Source: CAD feature listing. Evaluate the final solid. Frame: model axes, mm. A direction names the side the tool comes from. Round coordinates to 2 decimals unless told otherwise and drop trailing zeros. Write each loop counter-clockwise with the first axis right and the second up, starting at its lowest first coordinate (ties: lowest second). Pieces come first, ordered by that corner, then holes.
Autodesk Fusion 360 part; units mm, degrees
sketch "Sketch1" plane through (0, 0, 0) normal (0, 0, 1) x (1, 0, 0)
  line L0 (-42.9734, 5.15) -> (-45.9467, 0)
  line L1 (-45.9467, 0) -> (-42.9734, -5.15)
  line L2 (-42.9734, -5.15) -> (-37.0266, -5.15)
  line L3 (-37.0266, -5.15) -> (-34.0533, 0)
  line L4 (-34.0533, 0) -> (-37.0266, 5.15)
  line L5 (-37.0266, 5.15) -> (-42.9734, 5.15)
  line L6 (46, 5.15) -> (34, 5.15)
  line L7 (34, 5.15) -> (34, -5.15)
  line L8 (34, -5.15) -> (46, -5.15)
  line L9 (46, 5.15) -> (34, -5.15) construction
  line L10 (34, 5.15) -> (46, -5.15) construction
  line L11 (-32.8586, 7) -> (22.9763, 7)
  arc A0 (-32.8586, 7) -> (-32.8586, -7) centre (-40, 0) ccw
  arc A1 (22.9763, -7) -> (46, -5.15) centre (34, 0) ccw
  arc A2 (46, 5.15) -> (22.9763, 7) centre (34, 0) ccw
  line L12 (-32.8586, -7) -> (22.9763, -7)
  point P0 (-40, 0)
  point P1 (40, 0)
  dimension "d1" = 80
  dimension "d2" = 5.15
  dimension "d3" = 20
  dimension "d4" = 12
  dimension "d5" = 10.3
sketch "Sketch2" plane through (0, 0, 0) normal (0, 0, 1) x (1, 0, 0)
extrude "Extrude1" add sketch "Sketch1" along normal blind 4
fillet "Fillet1" radius 5 4 edges at (-32.8586, -7, 2) (22.9763, -7, 2) (22.9763, 7, 2) (-32.8586, 7, 2)
sketch "Sketch3" plane through (0, 0, 4) normal (0, 0, 1) x (1, 0, 0)
  line L0 (-42.9734, 5.15) -> (-37.0266, 5.15)
  line L1 (-37.0266, 5.15) -> (-34.0533, 0)
  line L2 (-34.0533, 0) -> (-37.0266, -5.15)
  line L3 (-37.0266, -5.15) -> (-42.9734, -5.15)
  line L4 (-42.9734, -5.15) -> (-45.9467, 0)
  line L5 (-45.9467, 0) -> (-42.9734, 5.15)
  arc A0 (-34, 8) -> (-34, -8) centre (-40, 0) ccw
  arc A1 (-31, -7) -> (-34, -8) centre (-31, -12) ccw
  line L6 (-31, -7) -> (20.5053, -7)
  arc A2 (24.2417, -8.6775) -> (20.5053, -7) centre (20.5053, -12) ccw
  arc A3 (24.2417, -8.6775) -> (46, -5.15) centre (34, 0) ccw
  line L7 (46, -5.15) -> (34, -5.15)
  line L8 (34, -5.15) -> (34, 5.15)
  line L9 (34, 5.15) -> (46, 5.15)
  arc A4 (46, 5.15) -> (24.2417, 8.6775) centre (34, 0) ccw
  arc A5 (20.5053, 7) -> (24.2417, 8.6775) centre (20.5053, 12) ccw
  line L10 (20.5053, 7) -> (-31, 7)
  arc A6 (-34, 8) -> (-31, 7) centre (-31, 12) ccw
  line L11 (-22.5, 2.5) -> (22.5, 2.5)
  line L12 (22.5, 2.5) -> (22.5, -2.5)
  line L13 (22.5, -2.5) -> (-22.5, -2.5)
  line L14 (-22.5, -2.5) -> (-22.5, 2.5)
  line L15 (-22.5, 2.5) -> (22.5, -2.5) construction
  line L16 (22.5, 2.5) -> (-22.5, -2.5) construction
  dimension "d11" = 45
  dimension "d12" = 5
extrude "Extrude2" cut sketch "Sketch3" against normal blind 1 contours L11 L12 L13 L14
sketch "Sketch4" plane through (0, 0, 4) normal (0, 0, 1) x (1, 0, 0)
  line L0 (22.5, 2.5) -> (22.5, -2.5)
  line L1 (22.5, -2.5) -> (-22.5, -2.5)
  line L2 (-22.5, -2.5) -> (-22.5, 2.5)
  line L3 (-22.5, 2.5) -> (22.5, 2.5)
  line L4 (-42.9734, 5.15) -> (-37.0266, 5.15)
  line L5 (-37.0266, 5.15) -> (-34.0533, 0)
  line L6 (-34.0533, 0) -> (-37.0266, -5.15)
  line L7 (-37.0266, -5.15) -> (-42.9734, -5.15)
  line L8 (-42.9734, -5.15) -> (-45.9467, 0)
  line L9 (-45.9467, 0) -> (-42.9734, 5.15)
  arc A0 (-34, 8) -> (-34, -8) centre (-40, 0) ccw
  arc A1 (-31, -7) -> (-34, -8) centre (-31, -12) ccw
  line L10 (-31, -7) -> (20.5053, -7)
  arc A2 (24.2417, -8.6775) -> (20.5053, -7) centre (20.5053, -12) ccw
  arc A3 (24.2417, -8.6775) -> (46, -5.15) centre (34, 0) ccw
  line L11 (46, -5.15) -> (34, -5.15)
  line L12 (34, -5.15) -> (34, 5.15)
  line L13 (34, 5.15) -> (46, 5.15)
  arc A4 (46, 5.15) -> (24.2417, 8.6775) centre (34, 0) ccw
  arc A5 (20.5053, 7) -> (24.2417, 8.6775) centre (20.5053, 12) ccw
  line L14 (20.5053, 7) -> (-31, 7)
  arc A6 (-34, 8) -> (-31, 7) centre (-31, 12) ccw
sketch "Sketch5" plane through (0, 0, 4) normal (0, 0, 1) x (1, 0, 0)
fillet "Fillet2" radius 2 4 edges at (-22.5, 2.5, 3.5) (-22.5, -2.5, 3.5) (22.5, 2.5, 3.5) (22.5, -2.5, 3.5)
fillet "Fillet3" radius 1 17 edges at (21.9142, 1.9142, 4) (22.5, 0, 4) (21.9142, -1.9142, 4) (0, -2.5, 4) (-21.9142, -1.9142, 4) (-22.5, 0, 4) (-21.9142, 1.9142, 4) (0, 2.5, 4) (36.0897, 12.8901, 4) (22.5531, 7.4386, 4) (-5.2473, 7, 4) (-32.5811, 7.2566, 4) (-50, 0, 4) (-32.5811, -7.2566, 4) (-5.2473, -7, 4) (22.5531, -7.4386, 4) (36.0897, -12.8901, 4)
Q1. Set-up query: faces 1 (the face through (-6, 7, 1)), 2 (the face through (0, 0, 3)), 3 (the face through (-32.56, -7.25, 1.52)), 4 (the face through (-35.56, -2.61, 1.97)). Return all of +Z, -Z, +X, -X, +Y, -Y with unobstructed straight access to the full face (end or side cutting, diameter ignored); none if empty.
Q2. Section query B-B, the plane x = -40. Output: boundary loops of the cut face in (y, z).
Q3. Mould query, pull axis X, two halves, no side actions, for faces 5 (the face through (-40, -5.15, 2)), 6 (the face through (-50, 0, 1)), 7 (the face through (34, 0, 2)), 8 (the face through (40, -5.15, 2)). Classes: pulls with the +X half, pulls with the -X half, needs draft (parallel to the pull), parting line crosses it, or undercut.
Q4. Pin query (flat end, axial travel): P1, Ø0.9, axis at x = 1.5, z = 1.5, coming from the +Y side; P2, Ø2, axis at x = 39.5, z = 2.5, coming from the -Y side; P3, Ø1.5, axis at x = -5.5, z = 1.5, coming from the -Y side. Return the tip coordinate at first contact, or that it passes through.
Q5. Section query A-A, the plane z = 1.5. Output: boundary loops of the cut face in (x, y), and give its area (3 significant figures).
Q6. Line query: line 1 (Y direction, x = -40, z = 2.4); line 2 (Y direction, x = -25, z = 1.2); line 3 (X direction, y = -1, z = 3.5). Output: solid intervals per line, ascending.
Filled in:
1. face 1: +Z, -Z, +Y
1. face 2: +Z
1. face 3: +Z, -Z, -Y
1. face 4: +Z, -Z
2. outline: (-10, 0) - (-5.15, 0) - (-5.15, 4) - (-9, 4) arc R1 ccw to (-10, 3) - close; (5.15, 0) - (10, 0) - (10, 3) arc R1 ccw to (9, 4) - (5.15, 4) - close
3. face 5: undercut
3. face 6: undercut
3. face 7: pulls with the +X half
3. face 8: needs draft
4. P1: stops at y = 7
4. P2: stops at y = -12.26
4. P3: stops at y = -7
5. outline: (-34, -8) arc R5 cw to (-31, -7) - (20.51, -7) arc R5 cw to (24.24, -8.68) arc R13.06 ccw to (46, -5.15) - (34, -5.15) - (34, 5.15) - (46, 5.15) arc R13.06 ccw to (24.24, 8.68) arc R5 cw to (20.51, 7) - (-31, 7) arc R5 cw to (-34, 8) arc R10 ccw (long way) to start; hole (-45.95, 0) - (-42.97, -5.15) - (-37.03, -5.15) - (-34.05, 0) - (-37.03, 5.15) - (-42.97, 5.15) - close
5. area: 1,360 mm2
6. line 1: y = -10 to -5.15, 5.15 to 10
6. line 2: y = -7 to 7
6. line 3: x = -49.82 to -45.37, -34.63 to -22.57, 22.57 to 34
